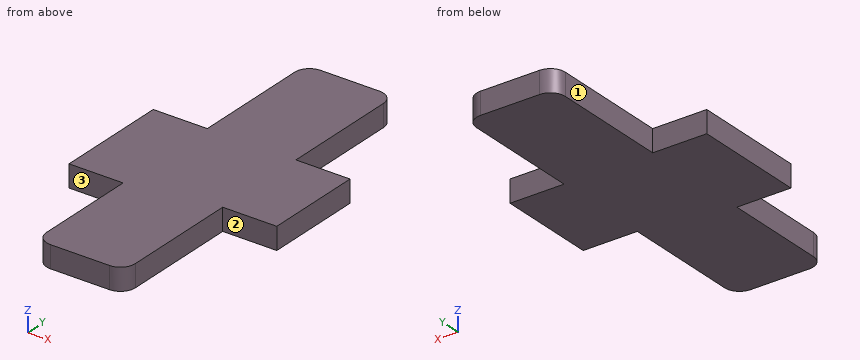
```python
from build123d import *

# Parameters (mm, degrees)
BASE_EXTRUDE_DEPTH = 3


with BuildPart() as part:
    # Sketch1 → Base-Extrude (new body)
    with BuildSketch(Plane.XY):
        with BuildLine():
            Line((-1588.329332145, -37.365903922), (-1588.329332145, -51.365903922))
            ThreePointArc((-1588.329332145, -51.365903922), (-1587.743545707, -52.780117485), (-1586.329332145, -53.365903922))
            Line((-1586.329332145, -53.365903922), (-1578.329332145, -53.365903922))
            ThreePointArc((-1578.329332145, -53.365903922), (-1576.915118583, -52.780117485), (-1576.329332145, -51.365903922))
            Line((-1576.329332145, -51.365903922), (-1576.329332145, -35.365903922))
            Line((-1576.329332145, -35.365903922), (-1569.009666147, -35.365903922))
            Line((-1569.009666147, -35.365903922), (-1569.009666147, -21.965903922))
            Line((-1569.009666147, -21.965903922), (-1576.329332145, -21.965903922))
            Line((-1576.329332145, -21.965903922), (-1576.329332145, -5.965903922))
            ThreePointArc((-1576.329332145, -5.965903922), (-1576.915118583, -4.55169036), (-1578.329332145, -3.965903922))
            Line((-1578.329332145, -3.965903922), (-1586.329332145, -3.965903922))
            ThreePointArc((-1586.329332145, -3.965903922), (-1587.743545707, -4.55169036), (-1588.329332145, -5.965903922))
            Line((-1588.329332145, -5.965903922), (-1588.329332145, -21.965903922))
            Line((-1588.329332145, -21.965903922), (-1595.648998143, -21.965903922))
            Line((-1595.648998143, -21.965903922), (-1595.648998143, -37.365903922))
            Line((-1595.648998143, -37.365903922), (-1588.329332145, -37.365903922))
        make_face()
    extrude(amount=BASE_EXTRUDE_DEPTH)


solid = part.part
```
The listing builds one solid part. Answer for the finished solid, in the listing's coordinates (mm). Face numbers are marked on the shaded views. A direction names the side the tool comes from. Coordinates: 2 decimals unless noted, no trailing zeros. Loops run counter-clockwise (first coordinate to the right, second up) from the corner with the lowest first, then second, coordinate; pieces in that order, holes last. Notation, with made-up numbers: M -25.5,14.25 L -1.5,14.25 A27 cw -1.5,46.25 Z; hole C 65,47.25 d1. An arc over 180 degrees is marked long. Answer as CSV lines item,"result". Start each with the question number.
(1) The part is cut by section C-C (x = -1591). Give the vertices of the cut face in (y, z).
(2) The part is cut by section B-B (y = -45). Give the vertices of the cut face in (x, z), and give its area (3 significant figures).
(3) The part is cut by section A-A (z = 2.35). Give the vertices of the cut face in (x, y), and give its area (3 significant figures).
(4) For the marked faces 1, 2 and 3, determine the directions among +Z, -Z, +X, -X, +Y, -Y from which every point of the face is accessible in a straight line to the end or side of a thin tool.
(5) Find the intervals of material crossed by L1, parallel to Y at x = -1571, z = 2.5; L2, parallel to X at y = -47.5, z = 1.6; L3, parallel to Y at x = -1590.25, z = 0.7, in increasing order. Write a range as [from, to].
(6) Given pin 1 (1.5 mm diameter, centred on x = -1571.5, z = 1, fed in from -Y); pin 2 (1.5 mm diameter, centred on x = -1592.5, z = 1, fed in from -Y); pin 3 (0.9 mm diameter, centred on x = -1571, z = 1.5, fed in from +Y), each flat-ended and moving along its own axis, determine where each tip first touches the part or whether it passes through.
Determined:
1,outline,"M -37.37,0 L -21.97,0 L -21.97,3 L -37.37,3 Z"
2,outline,"M -1588.33,0 L -1576.33,0 L -1576.33,3 L -1588.33,3 Z"
2,area,"36.0 mm2"
3,outline,"M -1595.65,-37.37 L -1588.33,-37.37 L -1588.33,-51.37 A2 ccw -1586.33,-53.37 L -1578.33,-53.37 A2 ccw -1576.33,-51.37 L -1576.33,-35.37 L -1569.01,-35.37 L -1569.01,-21.97 L -1576.33,-21.97 L -1576.33,-5.97 A2 ccw -1578.33,-3.97 L -1586.33,-3.97 A2 ccw -1588.33,-5.97 L -1588.33,-21.97 L -1595.65,-21.97 Z"
3,area,"800 mm2"
4,face 1,"+Z, -Z, -X, +Y"
4,face 2,"+Z, -Z, +X, -Y"
4,face 3,"+Z, -Z, -X, -Y"
5,L1,"[-35.37, -21.97]"
5,L2,"[-1588.33, -1576.33]"
5,L3,"[-37.37, -21.97]"
6,pin 1,"y = -35.37"
6,pin 2,"y = -37.37"
6,pin 3,"y = -21.97"
